Geometry: final body of the model. Coordinates: model frame, mm. A direction names the side the tool comes from. Round coordinates to 2 decimals unless told otherwise and drop trailing zeros. Order: outer loops, then holes, each group sorted by start corner. A loop starts at its lowest first (then second) coordinate and runs counter-clockwise, first axis right, second up. Notation, with made-up numbers: M -3,10 L 33,10 A15 cw 33,18 Z; hole C 9.5,-15.5 d11. An arc over 180 degrees is marked long. Put each result on its own line as item: value. Start each with the question number.
1) Section B-B, the plane y = -7.25. Return loops of the section in (x, z).
2) Draft query along Y for faces 6 (the flat face through (1, -25.5, 2)), 7 (the flat face through (0, -12, 5)), 8 (the flat face through (22, -12, 4)). Return one class per face: pulls with the +Y half, pulls with the -Y half, needs draft (parallel to the pull), parting line crosses it, or undercut.
3) First-contact query: P1, Ø4, axis at x = 18.5, z = 3.5, coming from the +Y side; P2, Ø1, axis at x = 12, y = -7, coming from the +Z side. Flat tips, straight axial feed; report the tip coordinate or a pass-through.
4) Access query for faces 1 (the flat face through (3, 1, 3)), 2 (the flat face through (3, -25, 3)), 3 (the flat face through (1, -24, 3)), 4 (the flat face through (21.5, -11.8, 8)), 5 (the flat face through (21, -12, 5)). Directions: +Z, -Z, +X, -X, +Y, -Y. A direction counts if a zero-diameter tool reaches every point of the face in a straight line with its end or side. Return the directions, or none.
5) Section D-D, the plane y = -10.25. Return loops of the section in (x, z).
6) Material intervals for probe 1 along X at (y, z) = (-10.75, 5); probe 2 along Y at (x, z) = (2.25, 3.5); probe 3 along Z at (x, y) = (0.25, -23.5), sorted ascending. Write a range as [from, to].
7) Section A-A, the plane z = 3. Return loops of the section in (x, y), then the cut area to 3 significant figures.
8) Section C-C, the plane x = 0.5. Return loops of the section in (y, z), then the cut area to 3 significant figures.
from build123d import *

# Parameters (mm, degrees)
F1_DEPTH = 8
F2_DEPTH = 2
F4_DEPTH = 1.5


with BuildPart() as f1:
    # F0 (on Top) → F1 (new body)
    with BuildSketch(Plane.XY):
        Polygon((0, -8), (0, 0), (-1, 0), (-1, -24), (0, -24), (0, -16), (0, -12), align=None)
    extrude(amount=F1_DEPTH)



with BuildPart() as f1b:
    # F0 (on Top) → F1, piece 2 (new body)
    with BuildSketch(Plane.XY):
        Polygon((22, 0), (21, 0), (21, -8), (21, -16), (21, -24), (22, -24), align=None)
    extrude(amount=F1_DEPTH)


with BuildPart() as f1_1:
    add(f1.part)

    add(f1b.part)  # F2 merges F1b
    # F0 (on Top) → F2 (join)
    with BuildSketch(Plane.XY):
        with BuildLine():
            Line((18, 0), (0, 0))
            Line((0, 0), (0, -8))
            Line((0, -8), (16.75, -8))
            ThreePointArc((16.75, -8), (17.1161165235, -7.1161165235), (18, -6.75))
            Line((18, -6.75), (18, 0))
        make_face()
        Polygon((0, -8), (0, 0), (-1, 0), (-1, -24), (0, -24), (0, -16), (0, -12), align=None)
        with BuildLine():
            Line((21, 0), (18, 0))
            Line((18, 0), (18, -6.75))
            ThreePointArc((18, -6.75), (18.8838834765, -7.1161165235), (19.25, -8))
            Line((19.25, -8), (21, -8))
            Line((21, -8), (21, 0))
        make_face()
        Polygon((22, 0), (21, 0), (21, -8), (21, -16), (21, -24), (22, -24), align=None)
        with BuildLine():
            Line((16.75, -16), (0, -16))
            Line((0, -16), (0, -24))
            Line((0, -24), (18, -24))
            Line((18, -24), (18, -17.25))
            ThreePointArc((18, -17.25), (17.1161165235, -16.8838834765), (16.75, -16))
        make_face()
        with BuildLine():
            Line((21, -24), (21, -16))
            Line((21, -16), (19.25, -16))
            ThreePointArc((19.25, -16), (18.8838834765, -16.8838834765), (18, -17.25))
            Line((18, -17.25), (18, -24))
            Line((18, -24), (21, -24))
        make_face()
        with BuildLine():
            Line((18, -12), (0, -12))
            Line((0, -12), (0, -16))
            Line((0, -16), (16.75, -16))
            ThreePointArc((16.75, -16), (17.1161165235, -15.1161165235), (18, -14.75))
            Line((18, -14.75), (18, -12))
        make_face()
        with BuildLine():
            Line((21, -16), (21, -8))
            Line((21, -8), (19.25, -8))
            ThreePointArc((19.25, -8), (18.8838834765, -8.8838834765), (18, -9.25))
            Line((18, -9.25), (18, -12))
            Line((18, -12), (18, -14.75))
            ThreePointArc((18, -14.75), (18.8838834765, -15.1161165235), (19.25, -16))
            Line((19.25, -16), (21, -16))
        make_face()
        with BuildLine():
            Line((16.75, -8), (0, -8))
            Line((0, -8), (0, -12))
            Line((0, -12), (18, -12))
            Line((18, -12), (18, -9.25))
            ThreePointArc((18, -9.25), (17.1161165235, -8.8838834765), (16.75, -8))
        make_face()
    extrude(amount=F2_DEPTH)

    # F3 (on face) → F4 (join)
    with BuildSketch(Plane.XZ.offset(24)):
        Polygon((4, 2), (0, 2), (0, 6), (-1, 7), (-1, 0), (6, 0), align=None)
        Polygon((0, 6), (0, 2), (4, 2), align=None)
    extrude(amount=F4_DEPTH)

    # F6: F1 across plane


with BuildPart() as f1_2:
    add(f1_1.part)
    add(f1_1.part.mirror(Plane.XZ.offset(12)))


solid = f1_2.part
Result sheet:
1. outline: M -1,0 L 17,0 L 17,2 L 0,2 L 0,8 L -1,8 Z; M 19,0 L 22,0 L 22,8 L 21,8 L 21,2 L 19,2 Z
2. face 6: pulls with the -Y half
2. face 7: undercut
2. face 8: needs draft
3. P1: stops at y = 0
3. P2: stops at z = 2
4. face 1: +Z, +X, +Y
4. face 2: +Z, +X, -Y
4. face 3: +Z
4. face 4: +Z, +X, -X, +Y, -Y
4. face 5: +Z, +Y, -Y
5. outline: M -1,0 L 22,0 L 22,8 L 21,8 L 21,2 L 0,2 L 0,8 L -1,8 Z
6. probe 1: x = [-1, 0], [21, 22]
6. probe 2: y = [-25.5, -24], [0, 1.5]
6. probe 3: z = [0, 2]
7. outline: M -1,-25.5 L 3,-25.5 L 3,-24 L 0,-24 L 0,0 L 3,0 L 3,1.5 L -1,1.5 Z; M 21,-24 L 22,-24 L 22,0 L 21,0 Z
7. area: 60.0 mm2
8. outline: M -25.5,0 L 1.5,0 L 1.5,5.5 L 0,5.5 L 0,2 L -24,2 L -24,5.5 L -25.5,5.5 Z
8. area: 64.5 mm2
